from build123d import *

# Parameters (mm, degrees)
SKETCH1_W           = 50.8
SKETCH1_H           = 50.8
SKETCH1_W_2         = 44.45
SKETCH1_H_2         = 44.45
BOSS_EXTRUDE1_DEPTH = 279.4
SKETCH2_R           = 25.4
CUT_EXTRUDE1_DEPTH  = 139.7


with BuildPart() as part:
    # Sketch1 → Boss-Extrude1 (new body)
    with BuildSketch(Plane.XY):
        Rectangle(SKETCH1_W, SKETCH1_H)
        Rectangle(SKETCH1_W_2, SKETCH1_H_2, mode=Mode.SUBTRACT)
    extrude(amount=BOSS_EXTRUDE1_DEPTH)

    # Sketch2 → Cut-Extrude1 (cut, symmetric)
    with BuildSketch(Plane(origin=(0, 0, 0), x_dir=(0, 0, -1), z_dir=(1, 0, 0))):
        Circle(SKETCH2_R)
    extrude(amount=CUT_EXTRUDE1_DEPTH, both=True, mode=Mode.SUBTRACT)


solid = part.part
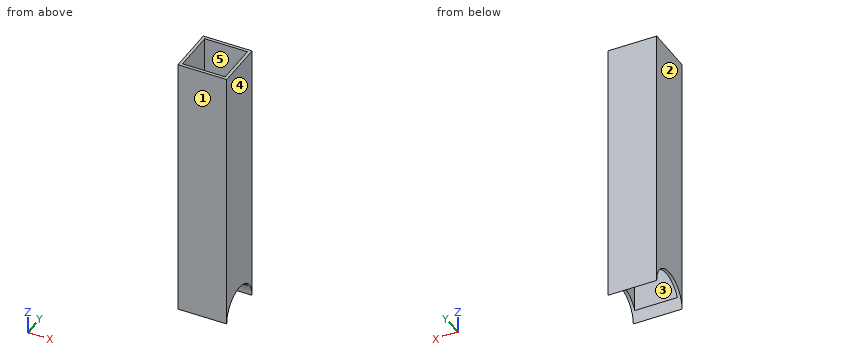
Design review of the part built by this model. Coordinates are the model's own, in mm. Face numbers are marked on the shaded views. A direction names the side the tool comes from. Coordinates: 2 decimals unless noted, no trailing zeros. Loops run counter-clockwise (first coordinate to the right, second up) from the corner with the lowest first, then second, coordinate; pieces in that order, holes last.
Item 1: Add section C-C (z = 216). Write out the cut boundary in (x, y) (3 decimals).
Completed:
outline: (-25.4, -25.4) - (25.4, -25.4) - (25.4, 25.4) - (-25.4, 25.4) - close; hole (-22.225, -22.225) - (22.225, -22.225) - (22.225, 22.225) - (-22.225, 22.225) - close
Item 2: For the marked faces 4 and 5, list the 3-axis set-ups (+Z, -Z, +X, -X, +Y, -Y) from which the entire face can be reached by the end or side of a thin tool; tool diameter is ignored.
Completed:
face 4: +Z, -Z, +X, +Y, -Y
face 5: +Z, -Z
Item 3: Wall thickness on L1, parallel to X at y = 14.5, z = 257 (3 decimals); L2, parallel to Z at x = -11, y = 22.5: over which ranges is each line inside the solid? List them lowest first.
Completed:
L1: x = -25.4 to -22.225, 22.225 to 25.4
L2: z = 11.79 to 279.4
Item 4: Draft analysis for pull direction Y (two halves, no side actions). For the marked faces 1, 2 and 3, state which applies: pulls with the +Y half, pulls with the -Y half, needs draft (parallel to the pull), parting line crosses it, or undercut.
Completed:
face 1: pulls with the -Y half
face 2: needs draft
face 3: undercut
Item 5: Add section A-A (y = 0). Write out the cut boundary in (x, z) (3 decimals).
Completed:
outline: (-25.4, 25.4) - (-22.225, 25.4) - (-22.225, 279.4) - (-25.4, 279.4) - close; (22.225, 25.4) - (25.4, 25.4) - (25.4, 279.4) - (22.225, 279.4) - close
Item 6: Add section B-B (x = 19). Write out the cut boundary in (y, z) (3 decimals), and give its area (3 significant figures).
Completed:
outline: (-25.4, 0) arc R25.4 cw to (-22.225, 12.297) - (-22.225, 279.4) - (-25.4, 279.4) - close; (22.225, 12.297) arc R25.4 cw to (25.4, 0) - (25.4, 279.4) - (22.225, 279.4) - close
area: 1,720 mm2
